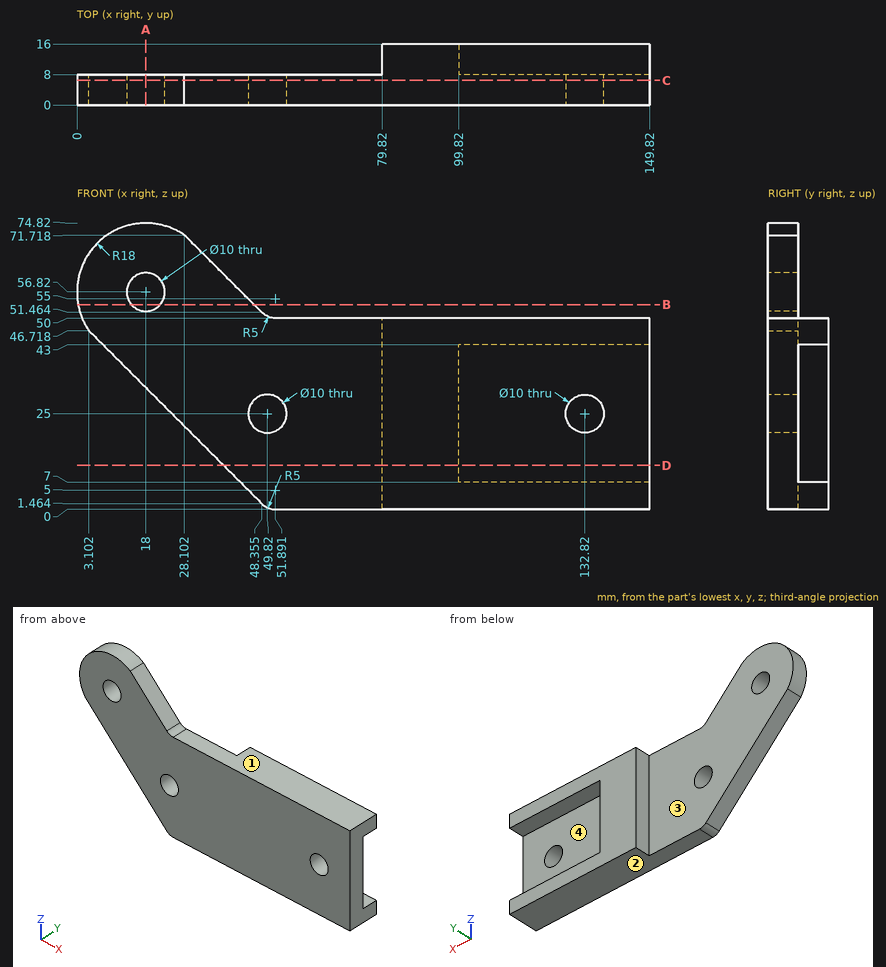
Drawing for the job (mm, zero at the part's lowest x, y, z). Round coordinates to 2 decimals unless told otherwise and drop trailing zeros. Loops run counter-clockwise (first coordinate to the right, second up) from the corner with the lowest first, then second, coordinate; pieces in that order, holes last. Notation, with made-up numbers: M 77,73 L 129,73 A26 ccw 129,103 Z; hole C 18.25,-6.75 d5. An arc over 180 degrees is marked long. Use a Markdown table: item, result. Add a question column.
(1) Cut at C-C (y = 6.5). Give the cut face in (x, z) (1 decimal).
(2) Pull direction Z, two halves, no side cores. Call the marked faces 1, 2, 3 and 4: +Z half, -Z half, draft (parallel to the pull), parting line (faces both ways), or undercut.
(3) Cut at D-D (z = 11.5). Give the cut face in (x, y), and give its area (3 significant figures).
(4) Cut at A-A (x = 18). Give the cut face in (y, z).
(5) Cut at B-B (z = 53.5). Give the cut face in (x, y), and give its area (3 significant figures).
(6) Drill centre lines: line 1 (Z direction, x = 130.5, y = 10.5); line 2 (Y direction, x = 22.5, z = 44.5); line 3 (X direction, y = 9, z = 6.5). Where is each one in solid material? Low to high.
(7) Flat gauge pins, fed straight in: pin 1 (12 mm diameter, centred on x = 119.5, z = 21, fed in from -Y); pin 2 (2.5 mm diameter, centred on y = 12.5, z = 21, fed in from +X); pin 3 (3 mm diameter, centred on y = 11.5, z = 16, fed in from -X); pin 4 (3 mm diameter, centred on x = 45.5, y = 8.5, fed in from +Z) (1 decimal). Where does each tip first touch, or does it go through?
Geometry says:
| question | item | result |
|---|---|---|
| 1 | outline | M 3.1,46.7 L 48.4,1.5 A5 ccw 51.9,0 L 149.8,0 L 149.8,50 L 51.9,50 A5 cw 48.4,51.5 L 28.1,71.7 A18 ccw Z; hole C 18,56.8 d10; hole C 49.8,25 d10; hole C 132.8,25 d10 |
| 2 | face 1 | +Z half |
| 2 | face 2 | -Z half |
| 2 | face 3 | draft |
| 2 | face 4 | undercut |
| 3 | outline | M 38.32,0 L 149.82,0 L 149.82,8 L 99.82,8 L 99.82,16 L 79.82,16 L 79.82,8 L 38.32,8 Z |
| 3 | area | 1,050 mm² |
| 4 | outline | M 0,31.82 L 8,31.82 L 8,51.82 L 0,51.82 Z; M 0,61.82 L 8,61.82 L 8,74.82 L 0,74.82 Z |
| 5 | outline | M 0.31,0 L 14.26,0 L 14.26,8 L 0.31,8 Z; M 21.74,0 L 46.32,0 L 46.32,8 L 21.74,8 Z |
| 5 | area | 308 mm² |
| 6 | line 1 | z = 0 to 7, 43 to 50 |
| 6 | line 2 | y = 0 to 8 |
| 6 | line 3 | x = 79.82 to 149.82 |
| 7 | pin 1 | stops at y = 0 |
| 7 | pin 2 | stops at x = 99.82 |
| 7 | pin 3 | stops at x = 79.82 |
| 7 | pin 4 | stops at z = 55.7 |
